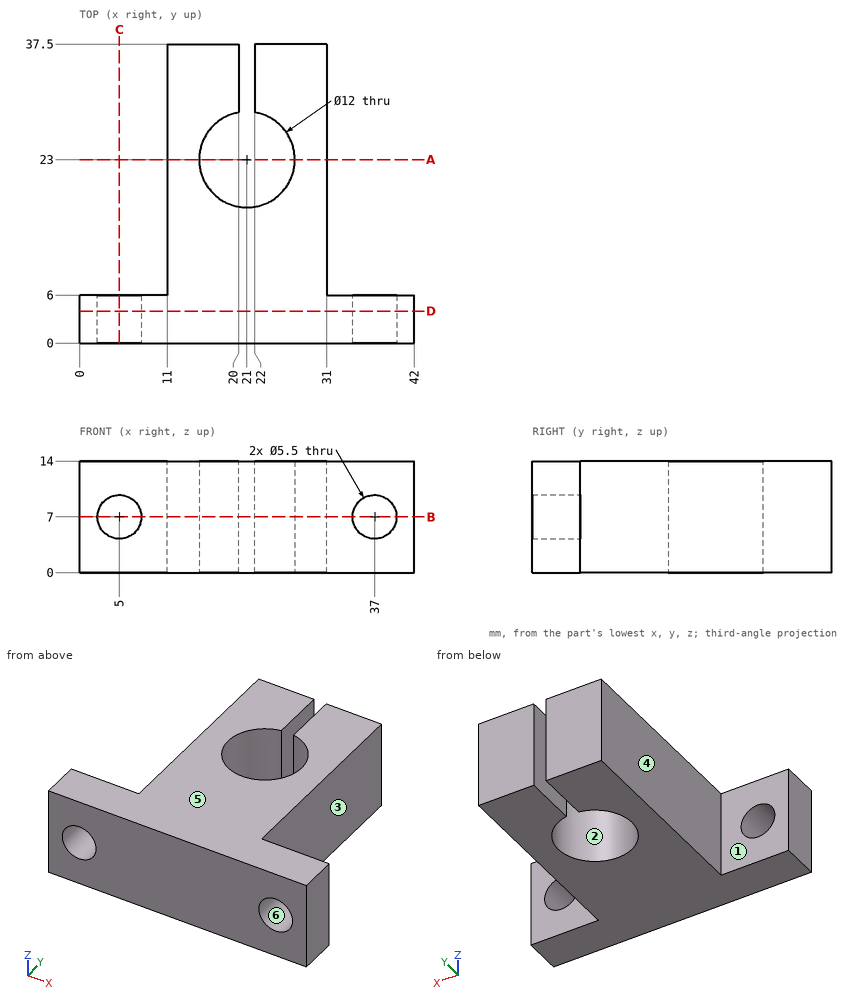
Geometry check sheet. Reference: drawing and pictorial views, mm from the part's lowest x, y, z. A direction names the side the tool comes from. Give positions to 0.01 mm unless a question says otherwise; leave off trailing zeros. Order: outer loops, then holes, each group sorted by start corner. A loop starts at its lowest first (then second) coordinate and runs counter-clockwise, first axis right, second up. Notation, with made-up numbers: (-20, 38) -> (-5, 38) arc R35 cw to (-5, 73) -> close; hole circle Ø9 at (51, 59.25). An arc over 180 degrees is marked (long way). Use CSV: the item, a comma, the result in double quotes. Start each with the question number.
1) Go/stop test with flat-tipped pins: P1, Ø3.5, axis at x = 5, z = 7, coming from the -Y side; P2, Ø7, axis at y = 25, z = 6.5, coming from the +X side; P3, Ø2.5, axis at y = 33, z = 8.5, coming from the -X side. Record where each tip stops, or that it passes through.
2) Sectioned sample at B-B, the plane z = 7. Record the boundary of the cut face in (x, y).
3) Material ranges on line 1 (X direction, y = 4.8, z = 7); line 2 (Z direction, x = 5, y = 2.7); line 3 (X direction, y = 23, z = 9.5), recorded low to high. Write a range as from..to.
4) Sectioned sample at A-A, the plane y = 23. Record the boundary of the cut face in (x, z).
5) Sectioned sample at C-C, the plane x = 5. Record the boundary of the cut face in (y, z), plus the area to 3 significant figures.
6) Mould release check, pull along Z, two halves, no side actions. Record for the marked faces 4, 5 and 6: released by +Z, released by -Z, zero draft, split by the parting line, or undercut.
7) Sectioned sample at D-D, the plane y = 4. Record the boundary of the cut face in (x, z).
8) Set-up check for the marked faces 1, 2 and 3: record each of +Z, -Z, +X, -X, +Y, -Y from which the full face is reachable in a straight line by a thin tool's end or side.
Recorded:
1,P1,"through"
1,P2,"x = 31"
1,P3,"x = 11"
2,outline,"(0, 0) -> (2.25, 0) -> (2.25, 6) -> (0, 6) -> close; (7.75, 0) -> (34.25, 0) -> (34.25, 6) -> (31, 6) -> (31, 37.5) -> (22, 37.5) -> (22, 28.92) arc R6 cw (long way) to (20, 28.92) -> (20, 37.5) -> (11, 37.5) -> (11, 6) -> (7.75, 6) -> close; (39.75, 0) -> (42, 0) -> (42, 6) -> (39.75, 6) -> close"
3,line 1,"0..2.25, 7.75..34.25, 39.75..42"
3,line 2,"0..4.25, 9.75..14"
3,line 3,"11..15, 27..31"
4,outline,"(11, 0) -> (15, 0) -> (15, 14) -> (11, 14) -> close; (27, 0) -> (31, 0) -> (31, 14) -> (27, 14) -> close"
5,outline,"(0, 0) -> (6, 0) -> (6, 4.25) -> (0, 4.25) -> close; (0, 9.75) -> (6, 9.75) -> (6, 14) -> (0, 14) -> close"
5,area,"51.0 mm2"
6,face 4,"zero draft"
6,face 5,"released by +Z"
6,face 6,"undercut"
7,outline,"(0, 0) -> (42, 0) -> (42, 14) -> (0, 14) -> close; hole circle Ø5.5 at (5, 7); hole circle Ø5.5 at (37, 7)"
8,face 1,"+Z, -Z, -X, +Y"
8,face 2,"+Z, -Z"
8,face 3,"+Z, -Z, +X, +Y"
